```python
from build123d import *

# Parameters (mm, degrees)
SKETCH1_R           = 8
BOSS_EXTRUDE1_DEPTH = 201
SKETCH2_R           = 0.828373934
SKETCH2_R_2         = 0.842670195
BOSS_EXTRUDE2_DEPTH = 20
BOSS_EXTRUDE3_DEPTH = 7.9
BOSS_EXTRUDE4_START = 10.4
SKETCH4_R           = 10.4
SKETCH4_R_2         = 8
BOSS_EXTRUDE4_DEPTH = 10.4


with BuildPart() as part:
    # Sketch1 → Boss-Extrude1 (new body)
    with BuildSketch(Plane(origin=(0, 0, 0), x_dir=(1, 0, 0), z_dir=(0, 1, 0))):
        with Locations(Location((0, 0, 0), (0, 0, 270))):
            Circle(SKETCH1_R)
    extrude(amount=BOSS_EXTRUDE1_DEPTH)

    # Sketch2 → Boss-Extrude2 (add)
    with BuildSketch(Plane(origin=(0, 201, 0), x_dir=(1, 0, 0), z_dir=(0, 1, 0))):
        with Locations(Location((-2.575042815, 0.066667775, 0), (0, 0, 270))):
            Circle(SKETCH2_R)
        with Locations(Location((2.750045724, 0.066667775, 0), (0, 0, 270))):
            Circle(SKETCH2_R_2)
    extrude(amount=BOSS_EXTRUDE2_DEPTH)

    # Sketch3 → Boss-Extrude3 (add)
    with BuildSketch(Plane(origin=(0, 201, 0), x_dir=(1, 0, 0), z_dir=(0, 1, 0))):
        Polygon((12.701705922, 0), (6.350852961, 11), (-6.350852961, 11), (-12.701705922, 0), (-6.350852961, -11), (6.350852961, -11), align=None)
    extrude(amount=-BOSS_EXTRUDE3_DEPTH)

    # Sketch4 → Boss-Extrude4 (add)
    with BuildSketch(Plane.XZ.offset(-193.1).offset(BOSS_EXTRUDE4_START)):
        with Locations(Location((0, 0, 0), (0, 0, 90))):
            Circle(SKETCH4_R)
        with Locations(Location((0, 0, 0), (0, 0, 270))):
            Circle(SKETCH4_R_2, mode=Mode.SUBTRACT)
    extrude(amount=-BOSS_EXTRUDE4_DEPTH)


solid = part.part
```
Design review of the part built by this model. Coordinates are the model's own, in mm. A direction names the side the tool comes from. Coordinates: 2 decimals unless noted, no trailing zeros. Order: outer loops, then holes, each group sorted by start corner. A loop starts at its lowest first (then second) coordinate and runs counter-clockwise, first axis right, second up. Notation, with made-up numbers: (37, 69.25) - (81, 69.25) arc R12 cw to (81, 75.25) - close; hole circle Ø11 at (-7.5, 34). An arc over 180 degrees is marked (long way). One line per question, with ' | ' between items.
Q1. To check wall thickness, follow line 1 along Y through (x, z) = (0, -4.5); line 2 along Y through (x, z) = (-5.25, 8.5); line 3 along X through (y, z) = (183, -2.5). State the ranges of each line that lie inside material, in increasing order.
Answer key:
line 1: y = 0 to 201 | line 2: y = 182.7 to 201 | line 3: x = -10.1 to 10.1
Q2. Consider section B-B, the plane y = 59. Give the boundary of the cut face in (x, z), then the cut area to 3 significant figures.
Answer key:
outline: circle Ø16 at (0, 0) | area: 201 mm2
Q3. Consider section A-A, the plane z = 4.25. Give the boundary of the cut face in (x, y).
Answer key:
outline: (-10.25, 193.1) - (-9.49, 193.1) - (-9.49, 182.7) - (-6.78, 182.7) - (-6.78, 0) - (6.78, 0) - (6.78, 182.7) - (9.49, 182.7) - (9.49, 193.1) - (10.25, 193.1) - (10.25, 201) - (-10.25, 201) - close
Q4. For faces 1 (the flat face through (4, 193.1, 10)), 2 (the flat face through (-9.571, 197.105, 5.423)), list the 3-axis set-ups (+Z, -Z, +X, -X, +Y, -Y) from which the entire face can be reached by the end or side of a thin tool; tool diameter is ignored.
Answer key:
face 1: -Y | face 2: +Z, -X, +Y, -Y
Q5. Clearance check with flat-ended pins moving along their axes: pin 1 Ø12 at (y, z) = (34, -2.5) entering from -X; pin 2 Ø6 at (x, y) = (9.5, 68) entering from -Z; pin 3 Ø1 at (x, z) = (0.5, 5.5) entering from +Y. State where each tip first meets the part, or that it passes through.
Answer key:
pin 1: stops at x = -8 | pin 2: stops at z = -4.66 | pin 3: stops at y = 201
